Source: CAD feature listing. Evaluate the final solid. Frame: model axes, mm. Face numbers are marked on the shaded views. A direction names the side the tool comes from. Coordinates: 2 decimals unless noted, no trailing zeros. Loops run counter-clockwise (first coordinate to the right, second up) from the corner with the lowest first, then second, coordinate; pieces in that order, holes last. Notation, with made-up numbers: (-18, -31) - (-9, -31) arc R21 cw to (-9, -13) - close; hole circle Ø2 at (-24, -33.75). An arc over 180 degrees is marked (long way). Write item = value, one per line. Start each with the question number.
from build123d import *

# Parameters (mm, degrees)
PAD_DEPTH       = 20
POCKET_DEPTH    = 5
POCKET001_DEPTH = 5
POCKET002_DEPTH = 10
POCKET003_DEPTH = 10
POCKET004_DEPTH = 10
POCKET005_DEPTH = 10
PAD001_DEPTH    = 2


with BuildPart() as part:
    # Sketch → Pad (new body)
    with BuildSketch(Plane.XY):
        Polygon((-10.136965, 24.465265), (9.95841, 24.465265), (19.936804, 9.913441), (9.95841, 0), (9.95841, -10.181935), (-9.998377, -10.181935), (-9.998377, 0), (-19.97677, 9.913441), align=None)
    extrude(amount=PAD_DEPTH)

    # Sketch001 (on Face10 of Pad) → Pocket (cut)
    with BuildSketch(Plane.XY.offset(20)):
        Polygon((-5.386747, 13.766779), (0, 13.766779), (-2.599782, 19.24781), align=None)
    extrude(amount=-POCKET_DEPTH, mode=Mode.SUBTRACT)

    # Sketch002 (on Face5 of Pocket) → Pocket001 (cut)
    with BuildSketch(Plane.XY.offset(20)):
        Polygon((1.335867, 14.164042), (6.583323, 14.671863), (3.87496, 19.919313), align=None)
    extrude(amount=-POCKET001_DEPTH, mode=Mode.SUBTRACT)

    # Sketch003 (on Face5 of Pocket001) → Pocket002 (cut)
    with BuildSketch(Plane.XY.offset(20)):
        Polygon((-6.538883, -0.90654), (-4.94164, -0.83048), (-4.561344, -8.816691), (-6.538883, -8.816691), align=None)
    extrude(amount=-POCKET002_DEPTH, mode=Mode.SUBTRACT)

    # Sketch004 (on Face5 of Pocket002) → Pocket003 (cut)
    with BuildSketch(Plane.XY.offset(20)):
        Polygon((-2.588899, -1.019739), (-1.067716, -1.019739), (-1.067716, -8.777773), (-2.588899, -9.00595), align=None)
    extrude(amount=-POCKET003_DEPTH, mode=Mode.SUBTRACT)

    # Sketch005 (on Face5 of Pocket003) → Pocket004 (cut)
    with BuildSketch(Plane.XY.offset(20)):
        Polygon((1.05956, -1.495936), (2.580743, -1.343817), (2.580743, -8.873672), (0.755325, -8.949731), align=None)
    extrude(amount=-POCKET004_DEPTH, mode=Mode.SUBTRACT)

    # Sketch006 (on Face5 of Pocket004) → Pocket005 (cut)
    with BuildSketch(Plane.XY.offset(20)):
        Polygon((5.072445, -1.486341), (6.878333, -1.486341), (6.878333, -9.145793), (5.072445, -9.33261), align=None)
    extrude(amount=-POCKET005_DEPTH, mode=Mode.SUBTRACT)

    # Sketch007 (on Face5 of Pocket005) → Pad001 (join)
    with BuildSketch(Plane.XY.offset(20)):
        Polygon((0, 10.495331), (-2.563093, 4.641765), (3.041384, 4.641765), align=None)
    extrude(amount=PAD001_DEPTH)


solid = part.part
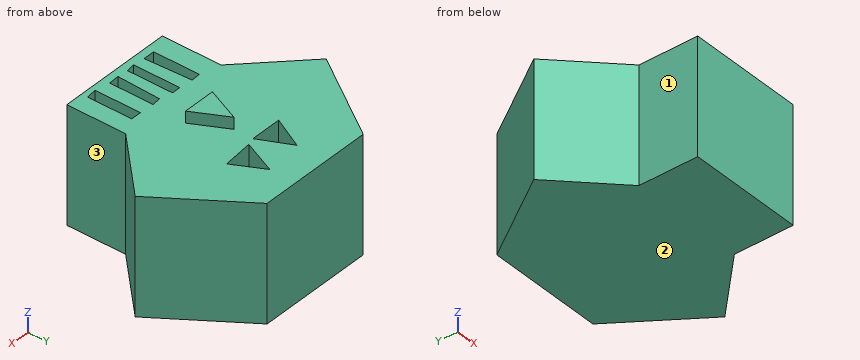
Item 1: First-contact query: pin 1 (5 mm diameter, centred on y = -5.5, z = 16.5, fed in from +X); pin 2 (4 mm diameter, centred on x = 4.5, y = 18, fed in from +Z); pin 3 (8 mm diameter, centred on y = -3.5, z = 12.5, fed in from +X). Flat tips, straight axial feed; report the tip coordinate or a pass-through.
Item 2: Cut plane A-A (z = 19.25). State how many separate pieces and enclosed holes the cut face has, then the cut area to 3 significant figures.
Item 3: Material intervals for L1, parallel to X at y = 18.5, z = 16; L2, parallel to X at y = 18, z = 18.5; L3, parallel to Z at x = -2, y = 15, sorted ascending. Write a range as [from, to].
Item 4: Cut plane C-C (z = 9). Return the cut outline in (x, y).
Item 5: Cut plane B-B (z = 14.25). Return the cut outline in (x, y).
Item 6: Cut plane D-D (x = 4.5). Return the cut outline in (y, z).
Item 7: Reachability of the marked faces 1, 2 and 3 from +Z, -Z, +X, -X, +Y, -Y: full face, straight path, thin tool, end or side. Return the list, or none.
Responses:
q1.pin_1 = 9.96
q1.pin_2 = 20
q1.pin_3 = 10.46
q2.separate_pieces = 1
q2.enclosed_holes = 6
q2.area = 855 mm2
q3.L1 = [-14.17, -2.98], [-2.25, 3.25], [4.61, 14.05]
q3.L2 = [-14.51, -3.23], [-2.01, 3.03], [4.87, 14.39]
q3.L3 = [0, 15]
q4.outline = (-19.98, 9.91) - (-10, 0) - (-10, -10.18) - (9.96, -10.18) - (9.96, 0) - (19.94, 9.91) - (9.96, 24.47) - (-10.14, 24.47) - close
q5.outline = (-19.98, 9.91) - (-10, 0) - (-10, -10.18) - (9.96, -10.18) - (9.96, 0) - (19.94, 9.91) - (9.96, 24.47) - (-10.14, 24.47) - close; hole (-6.54, -8.82) - (-4.56, -8.82) - (-4.94, -0.83) - (-6.54, -0.91) - close; hole (-2.59, -9.01) - (-1.07, -8.78) - (-1.07, -1.02) - (-2.59, -1.02) - close; hole (0.76, -8.95) - (2.58, -8.87) - (2.58, -1.34) - (1.06, -1.5) - close; hole (5.07, -9.33) - (6.88, -9.15) - (6.88, -1.49) - (5.07, -1.49) - close
q6.outline = (-10.18, 0) - (24.47, 0) - (24.47, 20) - (18.71, 20) - (18.71, 15) - (14.47, 15) - (14.47, 20) - (-10.18, 20) - close
q7.face_1 = +Z, -Z, -X, -Y
q7.face_2 = -Z, +X, -X, +Y, -Y
q7.face_3 = +Z, -Z, +X, -Y
